Geometry check sheet. Reference: the model listing, model coordinates, mm. A direction names the side the tool comes from. Round coordinates to 2 decimals unless told otherwise and drop trailing zeros. Order: outer loops, then holes, each group sorted by start corner. A loop starts at its lowest first (then second) coordinate and runs counter-clockwise, first axis right, second up.
(1) Cross-section at D-D on x = 0. Enter the section's corners in (y, z), and give its area (3 significant figures).
(2) Thickness scan on L1, parallel to Y at x = 8.5, z = 501; L2, parallel to Z at x = -20.5, y = 20; L3, parallel to X at y = 1.5, z = 525. Record the ranges inside material, lowest first.
(3) Set-up check for faces 4 (the face through (-10.2, 15.3, 517.8)), 5 (the face through (-6.723, 1.521, 546.1)), 6 (the face through (-2.116, 5.736, 516.321)): record each of +Z, -Z, +X, -X, +Y, -Y from which the full face is reachable in a straight line by a thin tool's end or side.
(4) Cross-section at C-C on y = 8. Enter the section's corners in (x, z).
(5) Cross-section at A-A on x = 12. Enter the section's corners in (y, z).
(6) Draft check along X on faces 1 (the face through (16.431, 1.521, 484.016)), 2 (the face through (12.51, 1.48, 490.17)), 3 (the face through (0, 3, 499)). Enter one of: pulls with the +X half, pulls with the -X half, needs draft (parallel to the pull), parting line crosses it, or undercut.
(7) Cross-section at B-B on z = 545. Enter the section's corners in (x, y).
(8) Gauge pin test, flat ends, axial feed: P1, Ø12, axis at x = -10.5, y = 13, coming from the +Z side; P2, Ø4, axis at x = 20, z = 544.05, coming from the -Y side; P3, Ø10, axis at y = 7.5, z = 522, coming from the -X side; P4, Ø16, axis at x = 2.5, z = 500, coming from the +Y side. Record the tip position at first contact, or that the pin passes through.
from build123d import *

# Parameters (mm, degrees)
SKETCH_1_R          = 1.7
EXTRUDE_2_DEPTH     = 3
EXTRUDE_3_DEPTH     = 25
SKETCH_4_R          = 10
CUT_EXTRUDE_1_DEPTH = 10
CUT_EXTRUDE_2_DEPTH = 10
FILLET_1_R          = 5


with BuildPart() as part:
    # 草图1 → 凸台-拉伸2 (new body)
    with BuildSketch(Plane(origin=(0, 0, 0), x_dir=(1, 0, 0), z_dir=(0, 1, 0))):
        Polygon((-17.55770441, -482.808341248), (17.55770441, -482.808341248), (26.316406952, -549.377139365), (-26.316406952, -549.377139365), align=None)
        with Locations(Location((-20, -544.050368455, 0), (0, 0, 270))):
            Circle(SKETCH_1_R, mode=Mode.SUBTRACT)
        with Locations(Location((20, -544.050368455, 0), (0, 0, 270))):
            Circle(SKETCH_1_R, mode=Mode.SUBTRACT)
        with Locations(Location((0, -488.550368455, 0), (0, 0, 270))):
            Circle(SKETCH_1_R, mode=Mode.SUBTRACT)
        with Locations(Location((-12, -488.550368455, 0), (0, 0, 270))):
            Circle(SKETCH_1_R, mode=Mode.SUBTRACT)
        with Locations(Location((12, -488.550368455, 0), (0, 0, 270))):
            Circle(SKETCH_1_R, mode=Mode.SUBTRACT)
    extrude(amount=EXTRUDE_2_DEPTH)

    # 草图3 → 凸台-拉伸3 (add)
    with BuildSketch(Plane(origin=(0, 3, 0), x_dir=(1, 0, 0), z_dir=(0, 1, 0))):
        Polygon((21.767013545, -514.800368455), (-21.767013545, -514.800368455), (-22.161734621, -517.800368455), (22.161734621, -517.800368455), align=None)
    extrude(amount=EXTRUDE_3_DEPTH)

    # 草图4 → 切除-拉伸1 (cut)
    with BuildSketch(Plane.XY.offset(517.800368455)):
        with Locations((0.051445108, 15.498034667)):
            Circle(SKETCH_4_R)
    extrude(amount=-CUT_EXTRUDE_1_DEPTH, mode=Mode.SUBTRACT)

    # 草图5 → 切除-拉伸2 (cut)
    with BuildSketch(Plane(origin=(0, 3, 0), x_dir=(1, 0, 0), z_dir=(0, 1, 0))):
        Polygon((0, -549.377139365), (10, -549.377139365), (0, -539.377139365), (-10, -549.377139365), align=None)
    extrude(amount=-CUT_EXTRUDE_2_DEPTH, mode=Mode.SUBTRACT)

    # 圆角1
    fillet_1_edges = [part.edges().sort_by_distance(p)[0] for p in [
        (-17.55770441, 1.5, 482.808341248),
        (17.55770441, 1.5, 482.808341248),
        (26.316406952, 1.5, 549.377139365),
        (-26.316406952, 1.5, 549.377139365),
        (-21.964374083, 28, 516.300368455),
        (21.964374083, 28, 516.300368455),
        (0, 1.5, 539.377139365),
    ]]
    fillet(fillet_1_edges, radius=FILLET_1_R)


solid = part.part
Found:
1. outline: (0, 482.81) - (3, 482.81) - (3, 486.85) - (0, 486.85) - close; (0, 490.25) - (3, 490.25) - (3, 514.8) - (5.5, 514.8) - (5.5, 517.8) - (3, 517.8) - (3, 541.45) - (0, 541.45) - close; (25.5, 514.8) - (28, 514.8) - (28, 517.8) - (25.5, 517.8) - close
1. area: 181 mm2
2. L1: y = 0 to 3
2. L2: z = 514.8 to 517.8
2. L3: x = -23.11 to 23.11
3. face 4: +Z, +X, -X, +Y
3. face 5: +Z, +Y, -Y
3. face 6: +Z, -Z
4. outline: (-22.16, 517.8) - (-21.77, 514.8) - (-6.57, 514.8) - (-6.57, 517.8) - close; (6.67, 514.8) - (21.77, 514.8) - (22.16, 517.8) - (6.67, 517.8) - close
5. outline: (0, 482.81) - (3, 482.81) - (3, 486.85) - (0, 486.85) - close; (0, 490.25) - (3, 490.25) - (3, 514.8) - (28, 514.8) - (28, 517.8) - (3, 517.8) - (3, 549.38) - (0, 549.38) - close
6. face 1: pulls with the +X half
6. face 2: undercut
6. face 3: needs draft
7. outline: (-25.58, 0) - (-21.41, 0) - (-21.41, 3) - (-25.58, 3) - close; (-18.59, 0) - (-5.62, 0) - (-5.62, 3) - (-18.59, 3) - close; (5.62, 0) - (18.59, 0) - (18.59, 3) - (5.62, 3) - close; (21.41, 0) - (25.58, 0) - (25.58, 3) - (21.41, 3) - close
8. P1: stops at z = 517.8
8. P2: stops at y = 0
8. P3: stops at x = -23
8. P4: stops at y = 3
